Here's how the part is built. I have some questions about the finished solid (model axes, mm). A direction names the side the tool comes from. Round coordinates to 2 decimals unless told otherwise and drop trailing zeros. Loops run counter-clockwise (first coordinate to the right, second up) from the corner with the lowest first, then second, coordinate; pieces in that order, holes last. Notation, with made-up numbers: M 41,16 L 87,16 A24 cw 87,29 Z; hole C -10.75,88 d3. An arc over 180 degrees is marked long. Answer as a JSON object with one key per item and string values.
from build123d import *

# Parameters (mm, degrees)
ESQUISSE1_W        = 40
ESQUISSE1_H        = 44
ESQUISSE1_W_2      = 20
ESQUISSE1_H_2      = 20
BOSS_EXTRU_1_DEPTH = 10
ESQUISSE3_W        = 10
ESQUISSE3_H        = 10
BOSS_EXTRU_2_DEPTH = 15
D_GAGEMENT_M31_D   = 3.4
CONG_2_R           = 10
CONG_3_R           = 5


with BuildPart() as part:
    # Esquisse1 → Boss.-Extru.1 (new body)
    with BuildSketch(Plane.XY):
        with Locations((20, 22)):
            Rectangle(ESQUISSE1_W, ESQUISSE1_H)
        with Locations((20, 24)):
            Rectangle(ESQUISSE1_W_2, ESQUISSE1_H_2, mode=Mode.SUBTRACT)
    extrude(amount=BOSS_EXTRU_1_DEPTH)

    # Esquisse3 → Boss.-Extru.2 (add)
    with BuildSketch(Plane.XY.offset(10)):
        with Locations((35, 5)):
            Rectangle(ESQUISSE3_W, ESQUISSE3_H)
        with Locations((5, 5)):
            Rectangle(ESQUISSE3_W, ESQUISSE3_H)
    extrude(amount=BOSS_EXTRU_2_DEPTH)

    # Dégagement M31 (through all)
    with Locations(Plane(origin=(0, 10, 0), x_dir=(1, 0, 0), z_dir=(0, 1, 0))):
        with Locations((5, -20.5), (35, -20.5)):
            Hole(D_GAGEMENT_M31_D / 2)

    # Congé2
    cong_2_edges = [part.edges().sort_by_distance(p)[0] for p in [
        (0, 44, 5),
        (40, 44, 5),
    ]]
    fillet(cong_2_edges, radius=CONG_2_R)

    # Congé3
    # the kernel refuses this fillet: 5 mm, written as the material it adds along each edge
    with BuildSketch(Plane(origin=(40, 10, 10), x_dir=(0, 1, 0), z_dir=(-1, 0, 0)), Plane(origin=(30, 10, 10), x_dir=(-1, 0, 0), z_dir=(0, -1, 0))) as cong_3_piece_1:
        with BuildLine():
            CenterArc((CONG_3_R, -CONG_3_R), CONG_3_R, 90, 90)
            Line((0, -CONG_3_R), (0, 0))
            Line((0, 0), (CONG_3_R, 0))
        make_face()
    extrude(amount=10)
    with BuildSketch(Plane(origin=(0, 10, 10), x_dir=(0, 1, 0), z_dir=(1, 0, 0)), Plane(origin=(10, 10, 10), x_dir=(1, 0, 0), z_dir=(0, -1, 0))) as cong_3_piece_2:
        with BuildLine():
            CenterArc((CONG_3_R, CONG_3_R), CONG_3_R, 180, 90)
            Line((0, CONG_3_R), (0, 0))
            Line((0, 0), (CONG_3_R, 0))
        make_face()
    extrude(amount=10)
    with BuildSketch(Plane(origin=(30, 22.5, 10), x_dir=(-1, 0, 0), z_dir=(0, -1, 0))) as cong_3_piece_3a_section:
        with BuildLine():
            CenterArc((CONG_3_R, -CONG_3_R), CONG_3_R, 90, 90)
            Line((0, -CONG_3_R), (0, 0))
            Line((0, 0), (CONG_3_R, 0))
        make_face()
    cong_3_piece_3a = extrude(amount=22.5, mode=Mode.PRIVATE)
    cong_3_piece_3a = split(cong_3_piece_3a, bisect_by=Plane(origin=(28.868024429, 14, 11.131975571), z_dir=(0, -1, 0)), keep=Keep.TOP, mode=Mode.PRIVATE)
    cong_3_piece_3a = split(cong_3_piece_3a, bisect_by=Plane(origin=(28.868024429, 10, 11.131975571), z_dir=(0, 1, 0)), keep=Keep.TOP, mode=Mode.PRIVATE)
    with BuildSketch(Plane(origin=(40, 10, 10), x_dir=(0, 1, 0), z_dir=(-1, 0, 0))) as cong_3_piece_3b_section:
        with BuildLine():
            CenterArc((CONG_3_R, -CONG_3_R), CONG_3_R, 90, 90)
            Line((0, -CONG_3_R), (0, 0))
            Line((0, 0), (CONG_3_R, 0))
        make_face()
    cong_3_piece_3b = extrude(amount=22.5, mode=Mode.PRIVATE)
    cong_3_piece_3b = split(cong_3_piece_3b, bisect_by=Plane(origin=(30, 11.061263152, 11.15683257), z_dir=(-1, 0, 0)), keep=Keep.TOP, mode=Mode.PRIVATE)
    cong_3_piece_3b = split(cong_3_piece_3b, bisect_by=Plane(origin=(23.75, 14, 11.15683257), z_dir=(0, -1, 0)), keep=Keep.TOP, mode=Mode.PRIVATE)
    cong_3_piece_3 = cong_3_piece_3a & cong_3_piece_3b
    add(cong_3_piece_3)
    with BuildSketch(Plane(origin=(0, 10, 10), x_dir=(0, 1, 0), z_dir=(1, 0, 0))) as cong_3_piece_4a_section:
        with BuildLine():
            CenterArc((CONG_3_R, CONG_3_R), CONG_3_R, 180, 90)
            Line((0, CONG_3_R), (0, 0))
            Line((0, 0), (CONG_3_R, 0))
        make_face()
    cong_3_piece_4a = extrude(amount=22.5, mode=Mode.PRIVATE)
    cong_3_piece_4a = split(cong_3_piece_4a, bisect_by=Plane(origin=(10, 11.061263152, 11.15683257), z_dir=(1, 0, 0)), keep=Keep.TOP, mode=Mode.PRIVATE)
    cong_3_piece_4a = split(cong_3_piece_4a, bisect_by=Plane(origin=(16.25, 14, 11.15683257), z_dir=(0, -1, 0)), keep=Keep.TOP, mode=Mode.PRIVATE)
    with BuildSketch(Plane(origin=(10, 22.5, 10), x_dir=(1, 0, 0), z_dir=(0, -1, 0))) as cong_3_piece_4b_section:
        with BuildLine():
            CenterArc((CONG_3_R, CONG_3_R), CONG_3_R, 180, 90)
            Line((0, CONG_3_R), (0, 0))
            Line((0, 0), (CONG_3_R, 0))
        make_face()
    cong_3_piece_4b = extrude(amount=22.5, mode=Mode.PRIVATE)
    cong_3_piece_4b = split(cong_3_piece_4b, bisect_by=Plane(origin=(11.131975571, 14, 11.131975571), z_dir=(0, -1, 0)), keep=Keep.TOP, mode=Mode.PRIVATE)
    cong_3_piece_4b = split(cong_3_piece_4b, bisect_by=Plane(origin=(11.131975571, 10, 11.131975571), z_dir=(0, 1, 0)), keep=Keep.TOP, mode=Mode.PRIVATE)
    cong_3_piece_4 = cong_3_piece_4a & cong_3_piece_4b
    add(cong_3_piece_4)
    # the kernel refuses this fillet: 5 mm, written as the material it takes off along each edge
    with BuildSketch(Plane(origin=(40, -12.5, 25), x_dir=(0, 0, -1), z_dir=(0, 1, 0)), Plane(origin=(30, 22.5, 25), x_dir=(0, 0, -1), z_dir=(0, -1, 0))) as cong_3_2_piece_1:
        with BuildLine():
            CenterArc((CONG_3_R, CONG_3_R), CONG_3_R, 180, 90)
            Line((0, CONG_3_R), (0, 0))
            Line((0, 0), (CONG_3_R, 0))
        make_face()
    extrude(amount=35, mode=Mode.SUBTRACT)
    with BuildSketch(Plane(origin=(10, 22.5, 25), x_dir=(0, 0, -1), z_dir=(0, -1, 0)), Plane(origin=(0, -12.5, 25), x_dir=(0, 0, -1), z_dir=(0, 1, 0))) as cong_3_2_piece_2:
        with BuildLine():
            CenterArc((CONG_3_R, -CONG_3_R), CONG_3_R, 90, 90)
            Line((0, -CONG_3_R), (0, 0))
            Line((0, 0), (CONG_3_R, 0))
        make_face()
    extrude(amount=35, mode=Mode.SUBTRACT)


solid = part.part
Item 1: For P1, Ø11, axis at x = 34.5, z = 21, coming from the +Y side; P2, Ø3, axis at x = 20, y = 10.5, coming from the +Z side, each with a flat end and sliding along its axis, tell me the tip position at first contact or that it passes through.
Solution:
{"P1": "stops at y = 10", "P2": "stops at z = 10"}
Item 2: I want a section at D-D on y = 7. List the corners of the cut face in (x, z) for me.
Solution:
{"outline": "M 0,0 L 40,0 L 40,20 A5 ccw 30,20 L 30,15 A5 cw 25,10 L 15,10 A5 cw 10,15 L 10,20 A5 ccw 0,20 Z; hole C 5,20.5 d3.4; hole C 35,20.5 d3.4"}
Item 3: I want a section at A-A on y = 24. List the corners of the cut face in (x, z) for me, plus the area to 3 significant figures.
Solution:
{"outline": "M 0,0 L 10,0 L 10,10 L 0,10 Z; M 30,0 L 40,0 L 40,10 L 30,10 Z", "area": "200 mm2"}
Item 4: I want a section at C-C on z = 5.25. List the corners of the cut face in (x, y) for me.
Solution:
{"outline": "M 0,0 L 40,0 L 40,34 A10 ccw 30,44 L 10,44 A10 ccw 0,34 Z; hole M 10,14 L 30,14 L 30,34 L 10,34 Z"}
Item 5: For faces 4 (the face through (20, 34, 5)), 5 (the face through (20, 36, 10)), 6 (the face through (10, 5, 17)), 7 (the face through (20, 44, 5)), which set-ups out of +Z, -Z, +X, -X, +Y, -Y let a thin tool reach every point of the face, with its end or its side?
Solution:
{"face 4": "+Z, -Z", "face 5": "+Z, +X, -X, +Y", "face 6": "+Z, +Y, -Y", "face 7": "+Z, -Z, +X, -X, +Y"}
Item 6: We'd pull the mould along X, two halves only. Please class faces 1 (the face through (5.221, 4.93, 18.814)), 2 (the face through (37.15, 40.99, 5.07)), 3 (the face through (36, 10, 18.8)): +X half, -X half, draft (parallel to the pull), parting line (faces both ways), or undercut.
Solution:
{"face 1": "undercut", "face 2": "+X half", "face 3": "draft"}
Item 7: I want a section at B-B on x = 18. List the corners of the cut face in (y, z) for me.
Solution:
{"outline": "M 0,0 L 14,0 L 14,10 L 0,10 Z; M 34,0 L 44,0 L 44,10 L 34,10 Z"}
Item 8: If I drill on L1, parallel to X at y = 20, z = 2.5; L2, parallel to Z at x = 35, y = 3; L3, parallel to Y at x = 22.5, z = 3.5, over which ranges is the centre line in solid material (lowest first)? Write a range as from..to.
Solution:
{"L1": "x = 0..10, 30..40", "L2": "z = 0..18.8, 22.2..25", "L3": "y = 0..14, 34..44"}
